```python
from build123d import *


with BuildPart() as f1:
    # F0 (on Front) → F1 (revolve)
    with BuildSketch(Plane.XZ):
        with BuildLine():
            Line((6.228764, 0), (0, 0))
            Line((0, 0), (0, -1))
            Line((0, -1), (6.228764, -1))
            ThreePointArc((6.228764, -1), (8.286747, -0.182821), (9.223569, 1.823529))
            Line((9.223569, 1.823529), (10, 15))
            Line((10, 15), (26, 15))
            Line((26, 15), (26, 5))
            Line((26, 5), (27, 5))
            Line((27, 5), (27, 16))
            Line((27, 16), (9.057191, 16))
            Line((9.057191, 16), (8.225301, 1.882353))
            ThreePointArc((8.225301, 1.882353), (7.600753, 0.544786), (6.228764, 0))
        make_face()
    revolve(axis=Axis((0, 0, -0.5), (0, 0, 1)))


solid = f1.part
```
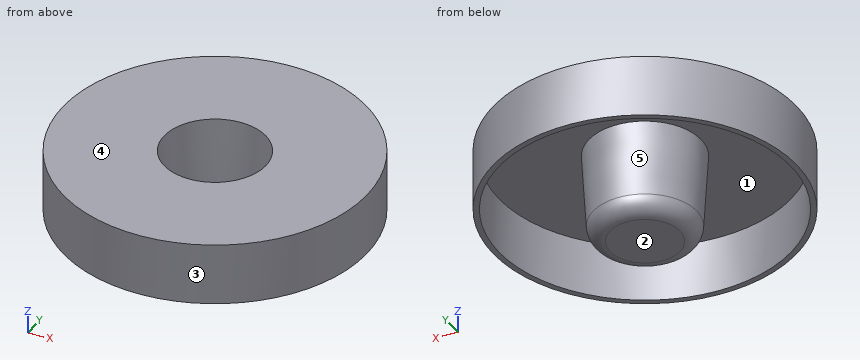
Check sheet for the modelled part. Datum: model origin and axes. Units: mm. Face numbers are marked on the shaded views. A direction names the side the tool comes from. Round coordinates to 2 decimals unless told otherwise and drop trailing zeros. Order: outer loops, then holes, each group sorted by start corner. A loop starts at its lowest first (then second) coordinate and runs counter-clockwise, first axis right, second up. Notation, with made-up numbers: (-20, 70.25) -> (33, 70.25) arc R15 cw to (33, 95.25) -> close; hole circle Ø7 at (10, 6). An arc over 180 degrees is marked (long way). One line per item, written item: value. Start each with the question number.
Q1. Cross-section at D-D (x = -16). Record the boundary of the cut face in (y, z), and give its area (3 significant figures).
Q2. Cross-section at C-C (z = 8.75). Record the boundary of the cut face in (x, y), and give its area (3 significant figures).
Q3. Set-up check for the marked faces 1 and 2: record each of +Z, -Z, +X, -X, +Y, -Y from which the full face is reachable in a straight line by a thin tool's end or side.
Q4. Cross-section at A-A (x = 0). Record the boundary of the cut face in (y, z).
Q5. Mould release check, pull along X, two halves, no side actions. Record for the marked faces 3, 4 and 5: pulls with the +X half, pulls with the -X half, needs draft (parallel to the pull), parting line crosses it, or undercut.
Q6. Gauge pin test, flat ends, axial feed: pin 1 Ø4 at (x, y) = (11, 16) entering from -Z; pin 2 Ø4 at (y, z) = (21.5, 8.5) entering from +X; pin 3 Ø6 at (x, y) = (0, -2.5) entering from +Z. Record the tip position at first contact, or that the pin passes through.
Q7. Thickness scan on line 1 (Y direction, x = -6, z = 8.25); line 2 (Y direction, x = -4, z = 12); line 3 (Y direction, x = -22, z = 8.75). Record the ranges inside material, lowest first.
Completed:
1. outline: (-21.75, 5) -> (-20.49, 5) -> (-20.49, 15) -> (20.49, 15) -> (20.49, 5) -> (21.75, 5) -> (21.75, 16) -> (-21.75, 16) -> close
1. area: 68.6 mm²
2. outline: circle Ø54 at (0, 0); circle Ø19.26 at (0, 0); hole circle Ø52 at (0, 0); hole circle Ø17.26 at (0, 0)
2. area: 224 mm²
3. face 1: -Z
3. face 2: -Z, +X, -X, +Y, -Y
4. outline: (-27, 5) -> (-26, 5) -> (-26, 15) -> (-10, 15) -> (-9.22, 1.82) arc R3 ccw to (-6.23, -1) -> (6.23, -1) arc R3 ccw to (9.22, 1.82) -> (10, 15) -> (26, 15) -> (26, 5) -> (27, 5) -> (27, 16) -> (9.06, 16) -> (8.23, 1.88) arc R2 cw to (6.23, 0) -> (-6.23, 0) arc R2 cw to (-8.23, 1.88) -> (-9.06, 16) -> (-27, 16) -> close
5. face 3: parting line crosses it
5. face 4: needs draft
5. face 5: undercut
6. pin 1: stops at z = 15
6. pin 2: stops at x = 18.67
6. pin 3: stops at z = 0
7. line 1: y = -26.32 to -25.3, -7.5 to -6.16, 6.16 to 7.5, 25.3 to 26.32
7. line 2: y = -26.7 to -25.69, -8.97 to -7.86, 7.86 to 8.97, 25.69 to 26.7
7. line 3: y = -15.65 to -13.86, 13.86 to 15.65
